Could you check a few things on this model? Use its own coordinates, in mm. A direction names the side the tool comes from. Give positions to 0.01 mm unless a question says otherwise; leave off trailing zeros. Loops run counter-clockwise (first coordinate to the right, second up) from the corner with the lowest first, then second, coordinate; pieces in that order, holes last. Notation, with made-up numbers: (-20, 75.25) -> (33, 75.25) arc R15 ccw to (33, 97.25) -> close; hole circle Ø6 at (48, -15). An arc over 180 degrees is marked (long way). Write item = value, one per line. Start each with the question number.
1) I need wall thicknesses on probe 1 along X at (y, z) = (-33.03, 2); probe 2 along Y at (x, z) = (22.75, 0.85); probe 3 along Z at (x, y) = (63, 27.5). Which ranges of each line are inside material? Lowest first, please. Write a range as from..to.
2) I want a section at A-A (x = 43.15). List the corners of the cut face in (y, z) for me.
3) I want a section at C-C (x = 15). List the corners of the cut face in (y, z) for me.
4) If we mould it in two halves opening along Y, with no side actions, what happens to faces 5 (the face through (69.97, 10.02, -8.22)), 6 (the face through (51, 32.73, -3)), 7 (the face through (65, -23, 2))? For each: +Y half, -Y half, draft (parallel to the pull), parting line (faces both ways), or undercut.
5) I'm going to push flat-ended pins straight in: pin 1 Ø1.5 at (y, z) = (7.5, -7.5) entering from -X (3 decimals); pin 2 Ø20 at (x, y) = (2.5, 10.5) entering from -Z; pin 3 Ø1 at (x, z) = (28.5, -0.5) entering from -Y. Where does each tip first touch, or does it pass through?
6) I want a section at D-D (y = 28). List the corners of the cut face in (x, z) for me, and give its area (3 significant figures).
7) I want a section at B-B (y = -16.5). List the corners of the cut face in (x, z) for me.
8) On a 3-axis mill with a long thin cutter (end or side, diameter ignored), from which of +Z, -Z, +X, -X, +Y, -Y can I reach the whole of each face in a straight line? I mean faces 1 (the face through (83, 20, 2)), 2 (the face through (0, 20, -1.15)), 3 (the face through (51, 39, 0)), 4 (the face through (0, 23, 1)). Say none if no direction works.
from build123d import *

# Parameters (mm, degrees)
SKETCH_2_W                       = 102.2634
SKETCH_2_H                       = 83
EXTRUDE_1_DEPTH                  = 4
SKETCH_4_W                       = 54.5268
SKETCH_4_H                       = 6
EXTRUDE_2_DEPTH                  = 1.15
SKETCH_5_W                       = 47.7366
SKETCH_5_H                       = 25.46
EXTRUDE_3_DEPTH                  = 6.25
SKETCH_6_R                       = 1.375
EXTRUDE_4_DEPTH                  = 4
SKETCH_7_W                       = 13.3866
SKETCH_7_H                       = 1.23
CUT_EXTRUDE_1_DEPTH              = 89.062832682
SKETCH_8_W                       = 13.3866
SKETCH_8_H                       = 16.5
CUT_EXTRUDE_3_DEPTH              = 89.062832682
SKETCH_9_W                       = 15
SKETCH_9_H                       = 83
EXTRUDE_5_DEPTH                  = 4
SKETCH_10_R                      = 0.5
CUT_EXTRUDE_4_DEPTH              = 102.143771435
PATTERN_LINEAR_1_COUNT           = 3
PATTERN_LINEAR_1_PITCH           = 3
PATTERN_LINEAR_2_COUNT           = 2
PATTERN_LINEAR_2_PITCH           = 44.5
PATTERN_LINEAR_2_COPY_1_SKETCH_R = 0.5
PATTERN_LINEAR_2_COPY_1_DEPTH    = 102.143771435
PATTERN_LINEAR_2_COPY_2_SKETCH_R = 0.5
PATTERN_LINEAR_2_COPY_2_DEPTH    = 102.143771435
SKETCH_12_R                      = 0.5
CUT_EXTRUDE_5_DEPTH              = 102.143771435
PATTERN_LINEAR_3_COUNT           = 5
PATTERN_LINEAR_3_PITCH           = 3.5
SKETCH_13_R                      = 0.5
CUT_EXTRUDE_6_DEPTH              = 102.143771435
SKETCH_14_W                      = 92.2634
SKETCH_14_H                      = 30
SKETCH_14_W_2                    = 15
SKETCH_14_H_2                    = 25
SKETCH_14_W_3                    = 54.5268
SKETCH_14_H_3                    = 22
CUT_EXTRUDE_7_DEPTH              = 102.143771435


with BuildPart() as part:
    # 草图2 → 凸台-拉伸1 (new body)
    with BuildSketch(Plane.XY):
        with Locations((23.8683, 3.5)):
            Rectangle(SKETCH_2_W, SKETCH_2_H)
    extrude(amount=EXTRUDE_1_DEPTH)

    # 草图4 → 凸台-拉伸2 (add)
    with BuildSketch(Plane(origin=(0, 0, 0), x_dir=(-1, 0, 0), z_dir=(0, 0, -1))):
        with Locations((0, 20)):
            Rectangle(SKETCH_4_W, SKETCH_4_H)
    extrude(amount=EXTRUDE_2_DEPTH)

    # 草图5 → 凸台-拉伸3 (add)
    with BuildSketch(Plane(origin=(0, 0, 0), x_dir=(-1, 0, 0), z_dir=(0, 0, -1))):
        with Locations((-51.1317, 20)):
            Rectangle(SKETCH_5_W, SKETCH_5_H)
    extrude(amount=EXTRUDE_3_DEPTH)

    # 草图6 → 凸台-拉伸4 (add)
    with BuildSketch(Plane(origin=(0, 0, -6.25), x_dir=(-1, 0, 0), z_dir=(0, 0, -1))):
        with Locations((-70, 31.355)):
            Circle(SKETCH_6_R)
        with Locations((-70, 8.645)):
            Circle(SKETCH_6_R)
        with Locations((-43.15, 8.645)):
            Circle(SKETCH_6_R)
        with Locations((-32.2634, 31.355)):
            Circle(SKETCH_6_R)
        with BuildLine():
            Line((-70, 32.73), (-71.375, 32.73))
            Line((-71.375, 32.73), (-71.375, 31.355))
            ThreePointArc((-71.375, 31.355), (-70.972271824, 32.327271824), (-70, 32.73))
        make_face()
        with BuildLine():
            Line((-68.625, 32.73), (-70, 32.73))
            ThreePointArc((-70, 32.73), (-69.027728176, 32.327271824), (-68.625, 31.355))
            Line((-68.625, 31.355), (-68.625, 32.73))
        make_face()
        with BuildLine():
            Line((-30.8884, 31.355), (-30.8884, 32.73))
            Line((-30.8884, 32.73), (-32.2634, 32.73))
            ThreePointArc((-32.2634, 32.73), (-31.291128176, 32.327271824), (-30.8884, 31.355))
        make_face()
        with BuildLine():
            Line((-32.2634, 32.73), (-33.6384, 32.73))
            Line((-33.6384, 32.73), (-33.6384, 31.355))
            ThreePointArc((-33.6384, 31.355), (-33.235671824, 32.327271824), (-32.2634, 32.73))
        make_face()
        with BuildLine():
            ThreePointArc((-70, 7.27), (-70.972271824, 7.672728176), (-71.375, 8.645))
            Line((-71.375, 8.645), (-71.375, 7.27))
            Line((-71.375, 7.27), (-70, 7.27))
        make_face()
        with BuildLine():
            Line((-68.625, 7.27), (-68.625, 8.645))
            ThreePointArc((-68.625, 8.645), (-69.027728176, 7.672728176), (-70, 7.27))
            Line((-70, 7.27), (-68.625, 7.27))
        make_face()
        with BuildLine():
            ThreePointArc((-41.775, 8.645), (-42.177728176, 7.672728176), (-43.15, 7.27))
            Line((-43.15, 7.27), (-41.775, 7.27))
            Line((-41.775, 7.27), (-41.775, 8.645))
        make_face()
        with BuildLine():
            Line((-44.525, 8.645), (-44.525, 7.27))
            Line((-44.525, 7.27), (-43.15, 7.27))
            ThreePointArc((-43.15, 7.27), (-44.122271824, 7.672728176), (-44.525, 8.645))
        make_face()
    extrude(amount=EXTRUDE_4_DEPTH)

    # 草图7 → 切除-拉伸1 (cut, through all)
    with BuildSketch(Plane(origin=(0, 0, -6.25), x_dir=(-1, 0, 0), z_dir=(0, 0, -1))):
        with Locations((-33.9567, 7.885)):
            Rectangle(SKETCH_7_W, SKETCH_7_H)
    extrude(amount=-CUT_EXTRUDE_1_DEPTH, mode=Mode.SUBTRACT)

    # 草图8 → 切除-拉伸3 (cut, through all)
    with BuildSketch(Plane(origin=(0, 0, 0), x_dir=(-1, 0, 0), z_dir=(0, 0, -1))):
        with Locations((-33.9567, 0.25)):
            Rectangle(SKETCH_8_W, SKETCH_8_H)
    extrude(amount=-CUT_EXTRUDE_3_DEPTH, mode=Mode.SUBTRACT)

    # 草图9 → 凸台-拉伸5 (add)
    with BuildSketch(Plane.XY):
        with Locations((82.5, 3.5)):
            Rectangle(SKETCH_9_W, SKETCH_9_H)
    extrude(amount=EXTRUDE_5_DEPTH)

    # 草图10 → 切除-拉伸4 (cut, through all)
    with BuildSketch(Plane(origin=(0, 0, 0), x_dir=(-1, 0, 0), z_dir=(0, 0, -1))):
        with Locations((-78.6, 8.47)):
            Circle(SKETCH_10_R)
        with Locations((-82.6, 8.47)):
            Circle(SKETCH_10_R)
    cut_extrude_4 = extrude(amount=-CUT_EXTRUDE_4_DEPTH, mode=Mode.SUBTRACT)

    # 阵列(线性)1: 切除-拉伸4 ×3
    with Locations(*[(0, i * PATTERN_LINEAR_1_PITCH, 0) for i in range(1, PATTERN_LINEAR_1_COUNT)]):
        add(cut_extrude_4, mode=Mode.SUBTRACT)

    # 阵列(线性)2: 切除-拉伸4 ×2
    with Locations(*[(0, -i * PATTERN_LINEAR_2_PITCH, 0) for i in range(1, PATTERN_LINEAR_2_COUNT)]):
        add(cut_extrude_4, mode=Mode.SUBTRACT)

    # 阵列(线性)2 copy 1 sketch → 阵列(线性)2 copy 1 (cut, through all)
    with BuildSketch(Plane(origin=(0, -41.5, 0), x_dir=(-1, 0, 0), z_dir=(0, 0, -1))):
        with Locations((-78.6, 8.47)):
            Circle(PATTERN_LINEAR_2_COPY_1_SKETCH_R)
        with Locations((-82.6, 8.47)):
            Circle(PATTERN_LINEAR_2_COPY_1_SKETCH_R)
    extrude(amount=-PATTERN_LINEAR_2_COPY_1_DEPTH, mode=Mode.SUBTRACT)

    # 阵列(线性)2 copy 2 sketch → 阵列(线性)2 copy 2 (cut, through all)
    with BuildSketch(Plane(origin=(0, -38.5, 0), x_dir=(-1, 0, 0), z_dir=(0, 0, -1))):
        with Locations((-78.6, 8.47)):
            Circle(PATTERN_LINEAR_2_COPY_2_SKETCH_R)
        with Locations((-82.6, 8.47)):
            Circle(PATTERN_LINEAR_2_COPY_2_SKETCH_R)
    extrude(amount=-PATTERN_LINEAR_2_COPY_2_DEPTH, mode=Mode.SUBTRACT)

    # 草图12 → 切除-拉伸5 (cut, through all)
    with BuildSketch(Plane(origin=(0, 0, 0), x_dir=(-1, 0, 0), z_dir=(0, 0, -1))):
        with Locations((-61.143527556, 41.241100687)):
            Circle(SKETCH_12_R)
        with Locations((-61.143527556, 37.741100687)):
            Circle(SKETCH_12_R)
    cut_extrude_5 = extrude(amount=-CUT_EXTRUDE_5_DEPTH, mode=Mode.SUBTRACT)

    # 阵列(线性)3: 切除-拉伸5 ×5
    with Locations(*[(-i * PATTERN_LINEAR_3_PITCH, 0, 0) for i in range(1, PATTERN_LINEAR_3_COUNT)]):
        add(cut_extrude_5, mode=Mode.SUBTRACT)

    # 草图13 → 切除-拉伸6 (cut, through all)
    with BuildSketch(Plane(origin=(0, 0, 0), x_dir=(-1, 0, 0), z_dir=(0, 0, -1))):
        with Locations((-22.75, -4.52)):
            Circle(SKETCH_13_R)
        with Locations((-18.125, -4.52)):
            Circle(SKETCH_13_R)
        with Locations((13.65, -4.52)):
            Circle(SKETCH_13_R)
        with Locations((18.27, -4.52)):
            Circle(SKETCH_13_R)
    extrude(amount=-CUT_EXTRUDE_6_DEPTH, mode=Mode.SUBTRACT)

    # 草图14 → 切除-拉伸7 (cut, through all)
    with BuildSketch(Plane(origin=(0, 0, 0), x_dir=(-1, 0, 0), z_dir=(0, 0, -1))):
        with Locations((-18.8683, -23)):
            Rectangle(SKETCH_14_W, SKETCH_14_H)
        with Locations((-82.5, 32.5)):
            Rectangle(SKETCH_14_W_2, SKETCH_14_H_2)
        with Locations((0, 34)):
            Rectangle(SKETCH_14_W_3, SKETCH_14_H_3)
    extrude(amount=-CUT_EXTRUDE_7_DEPTH, mode=Mode.SUBTRACT)


solid = part.part
Answer list:
q1.probe_1 = 65..78.1, 79.1..82.1, 83.1..90
q1.probe_2 = -8..-5.02, -4.02..23
q1.probe_3 = -6.25..4
q2.outline = (-8, 0) -> (7.27, 0) -> (7.27, -10.25) -> (10.02, -10.25) -> (10.02, -6.25) -> (32.73, -6.25) -> (32.73, 0) -> (45, 0) -> (45, 4) -> (-8, 4) -> close
q3.outline = (-8, 0) -> (17, 0) -> (17, -1.15) -> (23, -1.15) -> (23, 4) -> (-8, 4) -> close
q4.face_5 = undercut
q4.face_6 = +Y half
q4.face_7 = draft
q5.pin_1 = 41.775
q5.pin_2 = -1.15
q5.pin_3 = 8.5
q6.outline = (27.26, -6.25) -> (75, -6.25) -> (75, 4) -> (27.26, 4) -> close
q6.area = 489 mm^2
q7.outline = (65, 0) -> (90, 0) -> (90, 4) -> (65, 4) -> close
q8.face_1 = +Z, -Z, +X, +Y
q8.face_2 = -Z, -X, +Y, -Y
q8.face_3 = -Z, +X, -X, +Y
q8.face_4 = +Z, -Z, -X, +Y
